Design review of the part built by this model. Coordinates are the model's own, in mm. A direction names the side the tool comes from. Give positions to 0.01 mm unless a question says otherwise; leave off trailing zeros. Loops run counter-clockwise (first coordinate to the right, second up) from the corner with the lowest first, then second, coordinate; pieces in that order, holes last. Notation, with made-up numbers: (68.25, 56) - (123.25, 56) arc R31 cw to (123.25, 83) - close; hole circle Ø2 at (0.5, 13.5). An arc over 180 degrees is marked (long way). Put each result on its own line as item: value. Start each with the question number.
```python
from build123d import *

# Parameters (mm, degrees)
SKETCH2_W           = 138
SKETCH2_H           = 178
BOSS_EXTRUDE1_DEPTH = 5
SKETCH3_W           = 30
SKETCH3_H           = 3
CUT_EXTRUDE1_DEPTH  = 6
SKETCH4_W           = 30
SKETCH4_H           = 3
CUT_EXTRUDE2_DEPTH  = 8
SKETCH6_W           = 3
SKETCH6_H           = 38.70967742
CUT_EXTRUDE3_DEPTH  = 8
SKETCH5_W           = 3
SKETCH5_H           = 40
CUT_EXTRUDE4_DEPTH  = 8
SKETCH8_R           = 1.5
CUT_EXTRUDE5_DEPTH  = 6


with BuildPart() as part:
    # Sketch2 → Boss-Extrude1 (new body)
    with BuildSketch(Plane.XY):
        Rectangle(SKETCH2_W, SKETCH2_H)
    extrude(amount=BOSS_EXTRUDE1_DEPTH)

    # Sketch3 → Cut-Extrude1 (cut, through all)
    with BuildSketch(Plane.XY.offset(5)):
        with Locations((0, 82.5)):
            Rectangle(SKETCH3_W, SKETCH3_H)
    extrude(amount=-CUT_EXTRUDE1_DEPTH, mode=Mode.SUBTRACT)

    # Sketch4 → Cut-Extrude2 (cut)
    with BuildSketch(Plane.XY.offset(5)):
        with Locations((0, -82.5)):
            Rectangle(SKETCH4_W, SKETCH4_H)
    extrude(amount=-CUT_EXTRUDE2_DEPTH, mode=Mode.SUBTRACT)

    # Sketch6 → Cut-Extrude3 (cut)
    with BuildSketch(Plane.XY.offset(5)):
        with Locations((62.5, 0)):
            Rectangle(SKETCH6_W, SKETCH6_H)
    extrude(amount=-CUT_EXTRUDE3_DEPTH, mode=Mode.SUBTRACT)

    # Sketch5 → Cut-Extrude4 (cut)
    with BuildSketch(Plane.XY.offset(5)):
        with Locations((-62.5, 0)):
            Rectangle(SKETCH5_W, SKETCH5_H)
    extrude(amount=-CUT_EXTRUDE4_DEPTH, mode=Mode.SUBTRACT)

    # Sketch8 → Cut-Extrude5 (cut, through all)
    with BuildSketch(Plane.XY.offset(5)):
        with Locations((54, -74)):
            Circle(SKETCH8_R)
        with Locations((54, 74)):
            Circle(SKETCH8_R)
        with Locations((-54, 74)):
            Circle(SKETCH8_R)
        with Locations((-54, -74)):
            Circle(SKETCH8_R)
    extrude(amount=-CUT_EXTRUDE5_DEPTH, mode=Mode.SUBTRACT)


solid = part.part
```
Item 1: Consider section B-B (x = -12). State the section outline as (y, z) points, plus the area to 3 significant figures.
Item 2: For L1, parallel to Y at x = 54, z = 3.5; L2, parallel to Y at x = 11, z = 4.7; L3, parallel to X at y = -74, z = 3.2, list the stretches that pass through material, from the lowest coordinate up. Write a range as from..to.
Item 3: For P1, Ø8, axis at x = 42, y = -6.5, coming from the -Z side, flat-tipped, find the tip position at first contact; note if it passes through.
Item 4: Machinability: for faces 1 (the flat face through (-61, 0, 3)), 2 (the flat face through (-1, 1, 5)), which of the approach directions +Z, -Z, +X, -X, +Y, -Y give a long, thin tool a straight path to every point of the face, cutting with its end or side? Answer none if there is none.
Item 5: Consider section A-A (y = -6). State the section outline as (x, z) points, plus the area to 3 significant figures.
Item 6: Consider section C-C (z = 0.75). Count the separate pieces of the cut face and the enclosed holes in it, plus the area to 3 significant figures.
Geometry says:
1. outline: (-89, 0) - (-84, 0) - (-84, 5) - (-89, 5) - close; (-81, 0) - (81, 0) - (81, 5) - (-81, 5) - close; (84, 0) - (89, 0) - (89, 5) - (84, 5) - close
1. area: 860 mm2
2. L1: y = -89..-75.5, -72.5..72.5, 75.5..89
2. L2: y = -89..-84, -81..81, 84..89
2. L3: x = -69..-55.5, -52.5..52.5, 55.5..69
3. P1: stops at z = 0
4. face 1: +Z, -Z
4. face 2: +Z, +X, -X, +Y, -Y
5. outline: (-69, 0) - (-64, 0) - (-64, 5) - (-69, 5) - close; (-61, 0) - (61, 0) - (61, 5) - (-61, 5) - close; (64, 0) - (69, 0) - (69, 5) - (64, 5) - close
5. area: 660 mm2
6. separate pieces: 1
6. enclosed holes: 8
6. area: 24,100 mm2
